Work out the finished part from the listing and answer in its coordinate system (mm). A direction names the side the tool comes from. Coordinates: 2 decimals unless noted, no trailing zeros. Loops run counter-clockwise (first coordinate to the right, second up) from the corner with the lowest first, then second, coordinate; pieces in that order, holes last.
```python
from build123d import *

# Parameters (mm, degrees)
SKETCH1_W           = 144.5
SKETCH1_H           = 172.38
BOSS_EXTRUDE1_DEPTH = 35
SKETCH2_R           = 10.5
SKETCH2_R_2         = 1.99
CUT_EXTRUDE1_DEPTH  = 118.787005226
SKETCH3_R           = 15.25
CUT_EXTRUDE2_DEPTH  = 20
SKETCH4_W           = 32.5
SKETCH4_H           = 38
CUT_EXTRUDE3_DEPTH  = 5
SKETCH5_W           = 13.5
SKETCH5_H           = 7.5
CUT_EXTRUDE4_DEPTH  = 3
CUT_EXTRUDE5_DEPTH  = 80


with BuildPart() as part:
    # Sketch1 → Boss-Extrude1 (new body)
    with BuildSketch(Plane(origin=(0, 0, 0), x_dir=(1, 0, 0), z_dir=(0, 1, 0))):
        Rectangle(SKETCH1_W, SKETCH1_H)
    extrude(amount=BOSS_EXTRUDE1_DEPTH)

    # Sketch2 → Cut-Extrude1 (cut, through all)
    with BuildSketch(Plane.XZ):
        with Locations(Location((-42.25, -56.19, 0), (0, 0, 270))):
            Circle(SKETCH2_R)
        with Locations(Location((10.25, -56.19, 0), (0, 0, 270))):
            Circle(SKETCH2_R_2)
        with Locations(Location((42.25, -56.19, 0), (0, 0, 270))):
            Circle(SKETCH2_R)
        with Locations(Location((-10.25, 56.19, 0), (0, 0, 270))):
            Circle(SKETCH2_R_2)
        with Locations(Location((-42.25, 56.19, 0), (0, 0, 270))):
            Circle(SKETCH2_R)
        with Locations(Location((42.25, 56.19, 0), (0, 0, 270))):
            Circle(SKETCH2_R)
        Polygon((57.25, -20.94), (67.25, -20.94), (67.25, -17.44), (65.25, -17.44), (65.25, -17.94), (59.25, -17.94), (59.25, -17.44), (57.25, -17.44), align=None)
    extrude(amount=-CUT_EXTRUDE1_DEPTH, mode=Mode.SUBTRACT)

    # Sketch3 → Cut-Extrude2 (cut)
    with BuildSketch(Plane.XZ):
        with Locations(Location((-42.25, -56.19, 0), (0, 0, 270))):
            Circle(SKETCH3_R)
        with Locations(Location((42.25, -56.19, 0), (0, 0, 270))):
            Circle(SKETCH3_R)
        with Locations(Location((-42.25, 56.19, 0), (0, 0, 270))):
            Circle(SKETCH3_R)
        with Locations(Location((42.25, 56.19, 0), (0, 0, 270))):
            Circle(SKETCH3_R)
    extrude(amount=-CUT_EXTRUDE2_DEPTH, mode=Mode.SUBTRACT)

    # Sketch4 → Cut-Extrude3 (cut)
    with BuildSketch(Plane(origin=(0, 35, 0), x_dir=(1, 0, 0), z_dir=(0, 1, 0))):
        with Locations((-2.371711624, 0.554154498)):
            Rectangle(SKETCH4_W, SKETCH4_H)
    extrude(amount=-CUT_EXTRUDE3_DEPTH, mode=Mode.SUBTRACT)

    # Sketch5 → Cut-Extrude4 (cut)
    with BuildSketch(Plane(origin=(0, 35, 0), x_dir=(1, 0, 0), z_dir=(0, 1, 0))):
        with Locations((62.129216634, 19.25371769)):
            Rectangle(SKETCH5_W, SKETCH5_H)
    extrude(amount=-CUT_EXTRUDE4_DEPTH, mode=Mode.SUBTRACT)

    # Sketch6 → Cut-Extrude5 (cut)
    with BuildSketch(Plane.XZ):
        with BuildLine():
            Line((-1.305437085, -0.763536662), (-10.413111088, -9.871210665))
            ThreePointArc((-10.413111088, -9.871210665), (-10.413111088, -13.661303013), (-6.623018741, -13.661303013))
            Line((-6.623018741, -13.661303013), (7.01, -0.028284271))
            Line((7.01, -0.028284271), (-6.623018741, 13.60473447))
            ThreePointArc((-6.623018741, 13.60473447), (-10.413111088, 13.60473447), (-10.413111088, 9.814642123))
            Line((-10.413111088, 9.814642123), (-1.305437085, 0.706968119))
            ThreePointArc((-1.305437085, 0.706968119), (0.421531034, -0.028284271), (-1.305437085, -0.763536662))
        make_face()
    extrude(amount=-CUT_EXTRUDE5_DEPTH, mode=Mode.SUBTRACT)


solid = part.part
```
1. Straight lines are drawn through the part: probe 1 along X at (y, z) = (16, -17.5); probe 2 along Z at (x, y) = (42.5, 6.5); probe 3 along X at (y, z) = (18, 56). For each, find the intervals that lie inside material, in ascending order.
2. For faces 4 (the flat face through (-39, 20, 46)), 5 (the flat face through (-3, 33, 18.446)), 6 (the flat face through (62, 16, -17.94)), determine the directions among +Z, -Z, +X, -X, +Y, -Y from which every point of the face is accessible in a straight line to the end or side of a thin tool.
3. A cutting plane is placed at D-D, the plane z = 63. Give the vertices of the cut face in (x, y).
4. A cutting plane is placed at B-B, the plane y = 11. Count the separate pieces of the cut face and the enclosed holes in it, then the cut area to 3 significant figures.
5. A cutting plane is placed at A-A, the plane z = -56.19. Give the vertices of the cut face in (x, y), then the cut area to 3 significant figures.
6. A cutting plane is placed at C-C, the plane x = 42.25. Give the vertices of the cut face in (y, z).
7. Determine the mould class of faces 1 (the flat face through (72.25, 17, 1)), 2 (the cylindrical face through (38.23, 27.4, -65.89)), 3 (the flat face through (-17, 0, -1)) for opening direction X: released by +X, released by -X, zero draft, split by the parting line, or undercut.
Answers below:
1. probe 1: x = -72.25 to 57.25, 59.25 to 65.25, 67.25 to 72.25
1. probe 2: z = -86.19 to -71.44, -40.94 to 40.94, 71.44 to 86.19
1. probe 3: x = -72.25 to -57.5, -27 to -12.23, -8.27 to 27, 57.5 to 72.25
2. face 4: -Y
2. face 5: +Y
2. face 6: +Y, -Y
3. outline: (-72.25, 0) - (-55.9, 0) - (-55.9, 20) - (-50.24, 20) - (-50.24, 35) - (-72.25, 35) - close; (-34.26, 20) - (-28.6, 20) - (-28.6, 0) - (28.6, 0) - (28.6, 20) - (34.26, 20) - (34.26, 35) - (-34.26, 35) - close; (50.24, 20) - (55.9, 20) - (55.9, 0) - (72.25, 0) - (72.25, 35) - (50.24, 35) - close
4. separate pieces: 1
4. enclosed holes: 8
4. area: 21,700 mm2
5. outline: (-72.25, 0) - (-57.5, 0) - (-57.5, 20) - (-52.75, 20) - (-52.75, 35) - (-72.25, 35) - close; (-31.75, 20) - (-27, 20) - (-27, 0) - (8.26, 0) - (8.26, 35) - (-31.75, 35) - close; (12.24, 0) - (27, 0) - (27, 20) - (31.75, 20) - (31.75, 35) - (12.24, 35) - close; (52.75, 20) - (57.5, 20) - (57.5, 0) - (72.25, 0) - (72.25, 35) - (52.75, 35) - close
5. area: 3,070 mm2
6. outline: (0, -86.19) - (35, -86.19) - (35, -66.69) - (20, -66.69) - (20, -71.44) - (0, -71.44) - close; (0, -40.94) - (20, -40.94) - (20, -45.69) - (35, -45.69) - (35, 45.69) - (20, 45.69) - (20, 40.94) - (0, 40.94) - close; (0, 71.44) - (20, 71.44) - (20, 66.69) - (35, 66.69) - (35, 86.19) - (0, 86.19) - close
7. face 1: released by +X
7. face 2: undercut
7. face 3: zero draft
